```python
from build123d import *

# Parameters (mm, degrees)
EXTRUDE_1_DEPTH          = 85
SKETCH_2_R               = 58
EXTRUDE_2_DEPTH          = 5
SKETCH_3_R               = 40
CUT_EXTRUDE_1_DEPTH      = 44
SKETCH_4_R               = 35
CUT_EXTRUDE_2_DEPTH      = 187.38937738
PATTERN_CIRCULAR_1_COUNT = 6


with BuildPart() as part:
    # 草图1 → 凸台-拉伸1 (new body)
    with BuildSketch(Plane.XY):
        Polygon((0, 0), (-57, 0), (-57, 18), (-135, 18), (-135, 58), (-60, 58), (-60, 120), (60, 120), (60, 58), (135, 58), (135, 18), (57, 18), (57, 0), align=None)
    extrude(amount=-EXTRUDE_1_DEPTH)

    # 草图2 → 凸台-拉伸2 (add)
    with BuildSketch(Plane.XY):
        with Locations((0, 60)):
            Circle(SKETCH_2_R)
    extrude(amount=EXTRUDE_2_DEPTH)

    # 草图3 → 切除-拉伸1 (cut)
    with BuildSketch(Plane.XY.offset(5)):
        with Locations((0, 60)):
            Circle(SKETCH_3_R)
    extrude(amount=-CUT_EXTRUDE_1_DEPTH, mode=Mode.SUBTRACT)

    # 草图4 → 切除-拉伸2 (cut, through all)
    with BuildSketch(Plane.XY.offset(-39)):
        with Locations((0, 60)):
            Circle(SKETCH_4_R)
    extrude(amount=-CUT_EXTRUDE_2_DEPTH, mode=Mode.SUBTRACT)

    # 草图7 → M8 螺纹孔1 (revolve, cut)
    with BuildSketch(Plane(origin=(24, 101.569219382, 5), x_dir=(0, -1, 0), z_dir=(1, 0, 0))):
        Polygon((0, 0), (0, 29.802926105), (3.4, 27.76), (3.4, 0), align=None)
    hole_wizard_m8_1 = revolve(axis=Axis((24, 101.569219382, 11.35), (0, 0, -1)), mode=Mode.SUBTRACT)

    # 阵列(圆周)1: M8 螺纹孔1 ×6 about axis
    pattern_circular_1_axis = Axis((0, 60, 0), (0, 0, 1))
    for i in range(1, PATTERN_CIRCULAR_1_COUNT):
        add(hole_wizard_m8_1.rotate(pattern_circular_1_axis, i * 360 / PATTERN_CIRCULAR_1_COUNT), mode=Mode.SUBTRACT)


solid = part.part
```
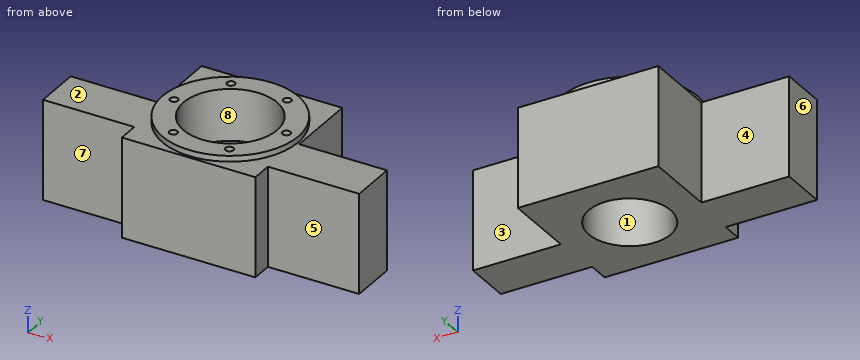
Can you work these out from the model? Positions are in its coordinate system, mm. Face numbers are marked on the shaded views. A direction names the side the tool comes from. Give positions to 0.01 mm unless a question says otherwise; leave off trailing zeros. Write each loop counter-clockwise with the first axis right and the second up, starting at its lowest first coordinate (ties: lowest second). Pieces come first, ordered by that corner, then holes. Notation, with made-up numbers: (77.5, -12) -> (90.5, -12) arc R23 ccw to (90.5, 27) -> close; hole circle Ø4 at (27.5, 68). An arc over 180 degrees is marked (long way). Write item = value, one per line.
(1) Thinking about a two-plate mould opening in X: for the marked faces 6, 7 and 8, which applies, released by +X, released by -X, zero draft, split by the parting line, or undercut?
Worked out:
face_6 = released by -X
face_7 = zero draft
face_8 = undercut
(2) I need wall thicknesses on probe 1 along X at (y, z) = (101, -19.5); probe 2 along Y at (x, z) = (21, -10.5); probe 3 along Y at (x, z) = (81, -49.5). Which ranges of each line are inside material? Lowest first, please. Write a range as from..to.
Worked out:
probe_1 = -60..-27.35, -20.65..20.65, 27.35..60
probe_2 = 0..16.83, 20.03..25.96, 94.04..99.97, 103.17..120
probe_3 = 18..58
(3) I'm going to push flat-ended pins straight in: P1, Ø1, axis at y = 74.5, z = -22.5, coming from the -X side; P2, Ø5.5, axis at x = -24, y = 18.43, coming from the +Z side; P3, Ø1.5, axis at x = -93.5, z = -51, coming from the +Y side. Where does each tip first touch, or does it pass through?
Worked out:
P1 = -60
P2 = -23.15
P3 = 58
(4) Suppose I cut it at A-A on z = -36. Write out the boundary of the cut face in (x, y), then the cut area to 3 significant figures.
Worked out:
outline = (-135, 18) -> (-57, 18) -> (-57, 0) -> (57, 0) -> (57, 18) -> (135, 18) -> (135, 58) -> (60, 58) -> (60, 120) -> (-60, 120) -> (-60, 58) -> (-135, 58) -> close; hole circle Ø80 at (0, 60)
area = 15,300 mm^2
(5) Suppose I cut it at D-D on z = -11. Write out the boundary of the cut face in (x, y), then the cut area to 3 significant figures.
Worked out:
outline = (-135, 18) -> (-57, 18) -> (-57, 0) -> (57, 0) -> (57, 18) -> (135, 18) -> (135, 58) -> (60, 58) -> (60, 120) -> (-60, 120) -> (-60, 58) -> (-135, 58) -> close; hole circle Ø6.8 at (-48, 60); hole circle Ø80 at (0, 60); hole circle Ø6.8 at (-24, 18.43); hole circle Ø6.8 at (-24, 101.57); hole circle Ø6.8 at (24, 18.43); hole circle Ø6.8 at (24, 101.57); hole circle Ø6.8 at (48, 60)
area = 15,000 mm^2
(6) Suppose I cut it at C-C on y = 44. Write out the boundary of the cut face in (x, z).
Worked out:
outline = (-135, -85) -> (-31.13, -85) -> (-31.13, -39) -> (-36.66, -39) -> (-36.66, 5) -> (-55.75, 5) -> (-55.75, 0) -> (-135, 0) -> close; (31.13, -85) -> (135, -85) -> (135, 0) -> (55.75, 0) -> (55.75, 5) -> (36.66, 5) -> (36.66, -39) -> (31.13, -39) -> close
(7) For the marked faces 1, 2, 3, 4 and 5, which set-ups out of +Z, -Z, +X, -X, +Y, -Y let a thin tool reach every point of the face, with its end or its side?
Worked out:
face_1 = +Z, -Z
face_2 = +Z
face_3 = +Z, -Z, +X, +Y
face_4 = +Z, -Z, -X, +Y
face_5 = +Z, -Z, +X, -Y
(8) Suppose I cut it at B-B on x = 0. Write out the boundary of the cut face in (y, z).
Worked out:
outline = (0, -85) -> (25, -85) -> (25, -39) -> (20, -39) -> (20, 5) -> (2, 5) -> (2, 0) -> (0, 0) -> close; (95, -85) -> (120, -85) -> (120, 0) -> (118, 0) -> (118, 5) -> (100, 5) -> (100, -39) -> (95, -39) -> close
